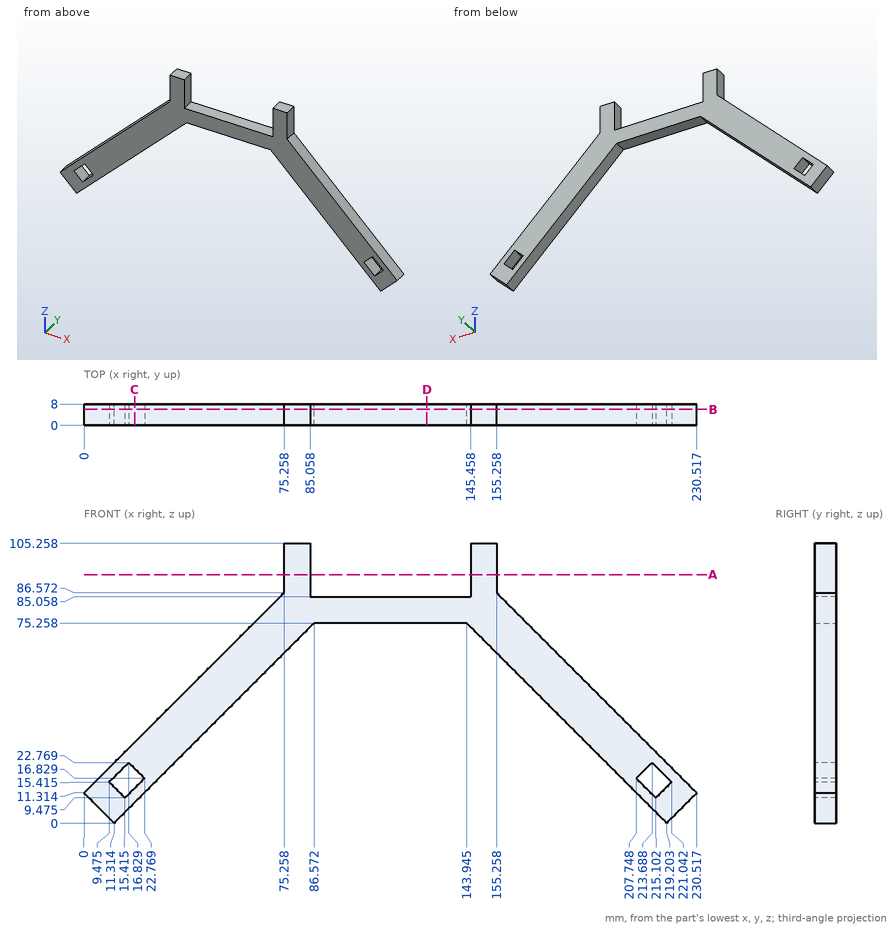
Drawing for the job (mm, zero at the part's lowest x, y, z). Round coordinates to 2 decimals unless told otherwise and drop trailing zeros. Write each loop counter-clockwise with the first axis right and the second up, starting at its lowest first coordinate (ties: lowest second). Pieces come first, ordered by that corner, then holes. Notation, with made-up numbers: (4, 71) - (42, 71) arc R16 ccw to (42, 77) - close; hole circle Ø4 at (-32.5, -1). An arc over 180 degrees is marked (long way). Write item = value, one per line. Start each with the question number.
Q1. Band-saw the part on C-C (x = 19). Give the cut face in (y, z), then the cut area to 3 significant figures.
Q2. Probe L1, parallel to X at y = 0.75, z = 99; L2, parallel to X at y = 0.75, z = 15 (1 decimal); L3, parallel to X at y = 2.25, z = 70 (1 decimal). List the from-to ranges inside material, lowest first. Write a range as from..to.
Q3. Band-saw the part on A-A (z = 93.5). Give the cut face in (x, y).
Q4. Band-saw the part on D-D (x = 129). Give the cut face in (y, z), then the cut area to 3 significant figures.
Q5. Drop flat-ended pins along their axis: pin 1 (3 mm diameter, centred on y = 6, z = 90, fed in from -X); pin 2 (2.5 mm diameter, centred on x = 111, y = 2.5, fed in from +Z); pin 3 (4 mm diameter, centred on x = 114.5, y = 2.5, fed in from -Z). Give the stop position or say it passes through.
Q6. Band-saw the part on B-B (y = 6). Give the cut face in (x, z) (1 decimal), then the cut area to 3 significant figures.
Answers below:
q1.outline = (0, 7.69) - (8, 7.69) - (8, 13.06) - (0, 13.06) - close; (0, 20.6) - (8, 20.6) - (8, 30.31) - (0, 30.31) - close
q1.area = 121 mm2
q2.L1 = 75.26..85.06, 145.46..155.26
q2.L2 = 3.7..9.9, 20.9..26.3, 204.2..209.6, 220.6..226.8
q2.L3 = 58.7..81.3, 149.2..171.8
q3.outline = (75.26, 0) - (85.06, 0) - (85.06, 8) - (75.26, 8) - close; (145.46, 0) - (155.26, 0) - (155.26, 8) - (145.46, 8) - close
q4.outline = (0, 75.26) - (8, 75.26) - (8, 85.06) - (0, 85.06) - close
q4.area = 78.4 mm2
q5.pin_1 = 75.26
q5.pin_2 = 85.06
q5.pin_3 = 75.26
q6.outline = (0, 11.3) - (11.3, 0) - (86.6, 75.3) - (143.9, 75.3) - (219.2, 0) - (230.5, 11.3) - (155.3, 86.6) - (155.3, 105.3) - (145.5, 105.3) - (145.5, 85.1) - (85.1, 85.1) - (85.1, 105.3) - (75.3, 105.3) - (75.3, 86.6) - close; hole (9.5, 15.4) - (15.4, 9.5) - (22.8, 16.8) - (16.8, 22.8) - close; hole (207.7, 16.8) - (215.1, 9.5) - (221, 15.4) - (213.7, 22.8) - close
q6.area = 4,280 mm2
